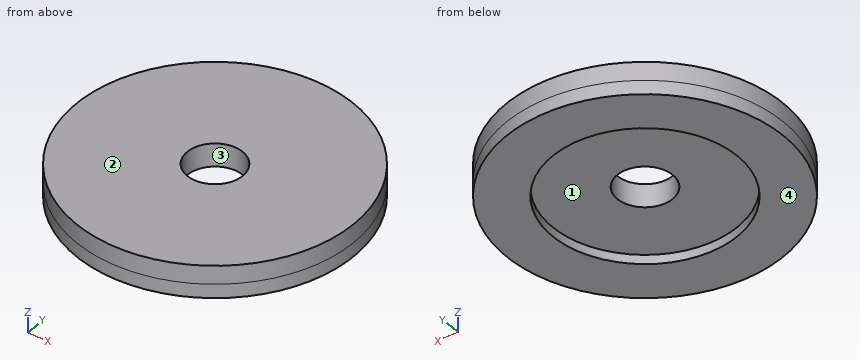
```python
from build123d import *

# Parameters (mm, degrees)
SKETCH2_R           = 30
BOSS_EXTRUDE1_DEPTH = 6
SKETCH3_R           = 8
CUT_EXTRUDE1_DEPTH  = 2
SKETCH4_R           = 6
CUT_EXTRUDE2_DEPTH  = 5
SKETCH5_R           = 30
SKETCH5_R_2         = 8
CUT_EXTRUDE3_DEPTH  = 2
BOSS_EXTRUDE3_START = 3
SKETCH7_R           = 30
SKETCH7_R_2         = 20
BOSS_EXTRUDE3_DEPTH = 3
BOSS_EXTRUDE4_START = 1
SKETCH8_R           = 20
SKETCH8_R_2         = 6
BOSS_EXTRUDE4_DEPTH = 1


with BuildPart() as part:
    # Sketch2 → Boss-Extrude1 (new body)
    with BuildSketch(Plane.XY):
        Circle(SKETCH2_R)
    extrude(amount=BOSS_EXTRUDE1_DEPTH)

    # Sketch3 → Cut-Extrude1 (cut)
    with BuildSketch(Plane(origin=(0, 0, 0), x_dir=(-1, 0, 0), z_dir=(0, 0, -1))):
        Circle(SKETCH3_R)
    extrude(amount=-CUT_EXTRUDE1_DEPTH, mode=Mode.SUBTRACT)

    # Sketch4 → Cut-Extrude2 (cut)
    with BuildSketch(Plane(origin=(0, 0, 2), x_dir=(-1, 0, 0), z_dir=(0, 0, -1))):
        Circle(SKETCH4_R)
    extrude(amount=-CUT_EXTRUDE2_DEPTH, mode=Mode.SUBTRACT)

    # Sketch5 → Cut-Extrude3 (cut)
    with BuildSketch(Plane(origin=(0, 0, 0), x_dir=(-1, 0, 0), z_dir=(0, 0, -1))):
        Circle(SKETCH5_R)
        Circle(SKETCH5_R_2, mode=Mode.SUBTRACT)
    extrude(amount=-CUT_EXTRUDE3_DEPTH, mode=Mode.SUBTRACT)

    # Sketch7 → Boss-Extrude3 (add)
    with BuildSketch(Plane(origin=(0, 0, 2), x_dir=(-1, 0, 0), z_dir=(0, 0, -1)).offset(BOSS_EXTRUDE3_START)):
        Circle(SKETCH7_R)
        Circle(SKETCH7_R_2, mode=Mode.SUBTRACT)
    extrude(amount=-BOSS_EXTRUDE3_DEPTH)

    # Sketch8 → Boss-Extrude4 (add)
    with BuildSketch(Plane(origin=(0, 0, 2), x_dir=(-1, 0, 0), z_dir=(0, 0, -1)).offset(BOSS_EXTRUDE4_START)):
        Circle(SKETCH8_R)
        Circle(SKETCH8_R_2, mode=Mode.SUBTRACT)
    extrude(amount=-BOSS_EXTRUDE4_DEPTH)


solid = part.part
```
Can you work these out from the model? Positions are in its coordinate system, mm. Face numbers are marked on the shaded views. A direction names the side the tool comes from. Round coordinates to 2 decimals unless told otherwise and drop trailing zeros. Loops run counter-clockwise (first coordinate to the right, second up) from the corner with the lowest first, then second, coordinate; pieces in that order, holes last.
Item 1: Will these pins go through, and if not, where does the flat tip stop? pin 1 Ø11 at (x, y) = (0, 0) entering from +Z (1 decimal); pin 2 Ø1 at (x, z) = (-21.5, 0.5) entering from +Y; pin 3 Ø10 at (x, y) = (5.5, 8) entering from -Z; pin 4 Ø4 at (y, z) = (11, 3) entering from -X.
Item 2: Please list where these lines run through material, in increasing order: L1, parallel to Y at x = 0, z = 0.4; L2, parallel to Y at x = 0, z = 3.2; L3, parallel to Z at x = 11.5, y = -7.5.
Item 3: Suppose I cut it at C-C, the plane z = 3.75. Write out the boundary of the cut face in (x, y).
Item 4: Which directions (+Z, -Z, +X, -X, +Y, -Y) give clear straight access to the entire face, cutting with the end or side of a thin tool? Please do the marked faces 1 and 2.
Item 5: Suppose I cut it at D-D, the plane x = -14. Write out the boundary of the cut face in (y, z), then the cut area to 3 significant figures.
Item 6: If we mould it in two halves opening along Y, with no side actions, what happens to the marked faces 3 and 4? For each: +Y half, -Y half, draft (parallel to the pull), parting line (faces both ways), or undercut.
Item 7: Suppose I cut it at A-A, the plane x = 0. Write out the boundary of the cut face in (y, z).
Reported:
1. pin 1: passes through
1. pin 2: stops at y = 21.42
1. pin 3: stops at z = 1
1. pin 4: stops at x = -28.62
2. L1: y = -30 to -20, 20 to 30
2. L2: y = -30 to -6, 6 to 30
2. L3: z = 1 to 6
3. outline: circle Ø60 at (0, 0); hole circle Ø12 at (0, 0)
4. face 1: -Z
4. face 2: +Z, +X, -X, +Y, -Y
5. outline: (-26.53, -1) - (-14.28, -1) - (-14.28, 1) - (14.28, 1) - (14.28, -1) - (26.53, -1) - (26.53, 6) - (-26.53, 6) - close
5. area: 314 mm2
6. face 3: undercut
6. face 4: draft
7. outline: (-30, -1) - (-20, -1) - (-20, 1) - (-6, 1) - (-6, 6) - (-30, 6) - close; (6, 1) - (20, 1) - (20, -1) - (30, -1) - (30, 6) - (6, 6) - close
